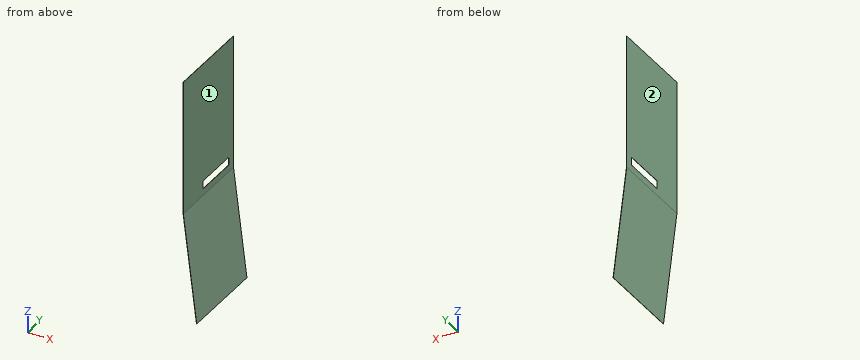
from build123d import *

# Parameters (mm, degrees)
BRIDA_BASE2_DEPTH          = 650
CORTAR_EXTRUIR1_DEPTH      = 1198.031165008
CORTAR_EXTRUIR1_DEPTH_BACK = 1198.031165008


# Sheet-metal steps are written as plain solids
with BuildPart() as part:
    # Croquis1 → Brida base2 (new body)
    with BuildSketch(Plane(origin=(0, 0, 0), x_dir=(1, 0, 0), z_dir=(0, 1, 0))):
        with BuildLine():
            Line((0, -1000), (0, -0.045297188))
            ThreePointArc((0, -0.045297188), (0.001388837, -8.5406e-05), (0.005550109, 0.044955885))
            Line((0.005550109, 0.044955885), (100, 810))
            Line((100, 810), (98.114316057, 810.232800487))
            Line((98.114316057, 810.232800487), (-1.880133834, 0.277756371))
            ThreePointArc((-1.880133834, 0.277756371), (-1.895028772, 0.116534721), (-1.9, -0.045297188))
            Line((-1.9, -0.045297188), (-1.9, -1000))
            Line((-1.9, -1000), (0, -1000))
        make_face()
    extrude(amount=BRIDA_BASE2_DEPTH)

    # Croquis11 → Cortar-Extruir1 (cut, two sides: drawn at the far end of the back side and taken through both)
    with BuildSketch(Plane.ZY.offset(1.9).offset(-CORTAR_EXTRUIR1_DEPTH_BACK)):
        with BuildLine():
            Line((60, 590), (100, 590))
            ThreePointArc((100, 590), (107.071067812, 587.071067812), (110, 580))
            Line((110, 580), (110, 265))
            ThreePointArc((110, 265), (107.071067812, 257.928932188), (100, 255))
            Line((100, 255), (60, 255))
            ThreePointArc((60, 255), (52.928932188, 257.928932188), (50, 265))
            Line((50, 265), (50, 580))
            ThreePointArc((50, 580), (52.928932188, 587.071067812), (60, 590))
        make_face()
    extrude(amount=CORTAR_EXTRUIR1_DEPTH + CORTAR_EXTRUIR1_DEPTH_BACK, mode=Mode.SUBTRACT)


solid = part.part
Check sheet for the modelled part. Datum: model origin and axes. Units: mm. Face numbers are marked on the shaded views. A direction names the side the tool comes from. Give positions to 0.01 mm unless a question says otherwise; leave off trailing zeros. Loops run counter-clockwise (first coordinate to the right, second up) from the corner with the lowest first, then second, coordinate; pieces in that order, holes last. Notation, with made-up numbers: M -14,-22 L 12,-22 A10 ccw 12,-9 Z; hole C 64,-0.75 d1. An arc over 180 degrees is marked long. Return JSON: item names as keys, results as strings. Group by question number.
1. Cross-section at B-B on y = 114. Record the boundary of the cut face in (x, z).
2. Tool access check on the marked faces 1 and 2. Record the directions out of +Z, -Z, +X, -X, +Y, -Y that give a thin tool (end or side, any length) a straight path to the whole face; none if there is none.
3. Cross-section at D-D on x = 28. Record the boundary of the cut face in (y, z), plus the area to 3 significant figures.
4. Cross-section at A-A on y = 420. Record the boundary of the cut face in (x, z).
5. Go/stop test with a flat-tipped pin: pin 1 (4 mm diameter, centred on y = 160.5, z = 326.5, fed in from +X). Record where the tip stops, or that it passes through.
6. Thickness scan on L1, parallel to X at y = 464, z = 565; L2, parallel to X at y = 139, z = -636.5. Record the ranges inside material, lowest first.
7. Cross-section at C-C on z = 424.5. Record the boundary of the cut face in (x, y), plus the area to 4 significant figures.
Return value:
{
 "1": {"outline": "M -1.9,0.05 A2.64 ccw -1.88,-0.28 L 98.11,-810.23 L 100,-810 L 0.01,-0.04 A0.74 cw 0,0.05 L 0,1000 L -1.9,1000 Z"},
 "2": {"face 1": "+Z, +X, +Y, -Y", "face 2": "+Z, -Z, -X, +Y, -Y"},
 "3": {"outline": "M 0,-242.31 L 650,-242.31 L 650,-226.8 L 0,-226.8 Z", "area": "10,100 mm^2"},
 "4": {"outline": "M -1.9,0.05 A2.64 ccw -1.88,-0.28 L 98.11,-810.23 L 100,-810 L 0.01,-0.04 A0.74 cw 0,0.05 L 0,50 L -1.9,50 Z; M -1.9,110 L 0,110 L 0,1000 L -1.9,1000 Z"},
 "5": {"pin 1": "x = 0"},
 "6": {"L1": "-1.9 to 0", "L2": "76.67 to 78.58"},
 "7": {"outline": "M -1.9,0 L 0,0 L 0,650 L -1.9,650 Z", "area": "1,235 mm^2"}
}
